Read the model definition and answer for the solid it produces. Units are mm, in the model's axes. Face numbers are marked on the shaded views. A direction names the side the tool comes from. Give positions to 0.01 mm unless a question says otherwise; leave off trailing zeros. Write each loop counter-clockwise with the first axis right and the second up, starting at its lowest first coordinate (ties: lowest second). Pieces come first, ordered by that corner, then holes. Notation, with made-up numbers: (-36.5, 77) -> (-29.5, 77) arc R21 cw to (-29.5, 95) -> close; hole circle Ø8 at (-29, 37.5). An arc over 180 degrees is marked (long way). Answer as CSV lines item,"result". Start each with the question number.
1. The part is cut by section C-C, the plane z = 0. Determine the outline of the cut face in (x, y), and give its area (3 significant figures).
2. Given pin 1 (2 mm diameter, centred on x = 22, z = 15, fed in from -Y); pin 2 (2.5 mm diameter, centred on y = 3, z = 0, fed in from +X); pin 3 (0.6 mm diameter, centred on y = -11, z = 8.5, fed in from -X), each flat-ended and moving along its own axis, determine where each tip first touches the part or whether it passes through.
3. Find the intervals of material crossed by line 1 (X direction, y = -4.75, z = 17); line 2 (Z direction, x = 1, y = -4.5); line 3 (Y direction, x = 18, z = 18), in increasing order.
4. A tool of negligible diameter and unlimited length cuts with its end or side. For the marked faces 1, 2, 3 and 4, from which of +Z, -Z, +X, -X, +Y, -Y can it reach the whole face along a straight path? Write none if from no direction.
5. The part is cut by section B-B, the plane y = -8.5. Determine the outline of the cut face in (x, z), and give its area (3 significant figures).
6. The part is cut by section A-A, the plane x = 0. Determine the outline of the cut face in (y, z).
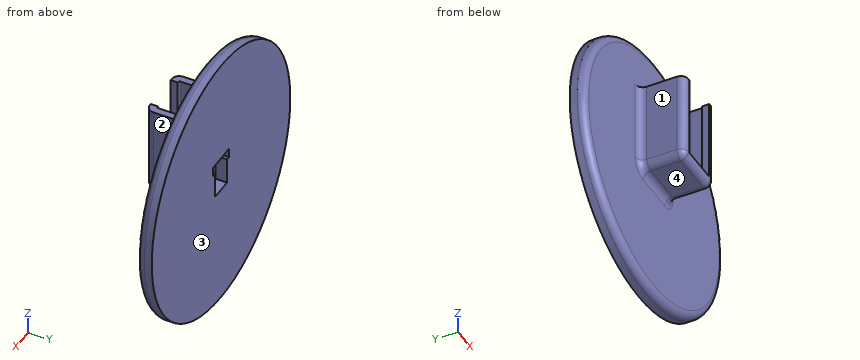
from build123d import *

# Parameters (mm, degrees)
SKETCH1_R                  = 35
ROUND_BODY_DEPTH           = 4
FILLET1_R                  = 2
SKETCH2_W                  = 6
SKETCH2_H                  = 7
SENSOR_SQUARE_HOLE_DEPTH   = 3
SKETCH4_W                  = 8
SKETCH4_H                  = 2.5
SENSOR_LEAD_HOLE_DEPTH     = 4
SKETCH5_W                  = 15
SKETCH5_H                  = 24
BACK_HOLDER_DEPTH          = 12
SKETCH6_W                  = 11.2
SKETCH6_H                  = 10.1
HOLDER_SLOT_DEPTH          = 22
HOLDER_ROUNDS_R            = 2
SKETCH7_W                  = 10
SKETCH7_H                  = 1.9
HOLDER_TOP_REMOVAL_DEPTH   = 22
HOLDER_MICRO_TOP_FILLETS_R = 0.5


with BuildPart() as part:
    # Sketch1 → Round Body (new body)
    with BuildSketch(Plane(origin=(0, 0, 0), x_dir=(1, 0, 0), z_dir=(0, 1, 0))):
        with Locations(Location((0, 0, 0), (0, 0, 270))):
            Circle(SKETCH1_R)
    extrude(amount=ROUND_BODY_DEPTH)

    # Fillet1
    fillet1_edges = [part.edges().sort_by_distance(p)[0] for p in [
        (0, 0, -35),
    ]]
    fillet(fillet1_edges, radius=FILLET1_R)

    # Sketch2 → Sensor Square Hole (cut)
    with BuildSketch(Plane(origin=(0, 4, 0), x_dir=(1, 0, 0), z_dir=(0, 1, 0))):
        with Locations((0, -1)):
            Rectangle(SKETCH2_W, SKETCH2_H)
    extrude(amount=-SENSOR_SQUARE_HOLE_DEPTH, mode=Mode.SUBTRACT)

    # Sketch4 → Sensor Lead Hole (cut)
    with BuildSketch(Plane(origin=(0, 4, 0), x_dir=(1, 0, 0), z_dir=(0, 1, 0))):
        with Locations((0, -5.75)):
            Rectangle(SKETCH4_W, SKETCH4_H)
    extrude(amount=-SENSOR_LEAD_HOLE_DEPTH, mode=Mode.SUBTRACT)

    # Sketch5 → Back Holder (add)
    with BuildSketch(Plane.XZ):
        with Locations((0, 9)):
            Rectangle(SKETCH5_W, SKETCH5_H)
    extrude(amount=BACK_HOLDER_DEPTH)

    # Sketch6 → Holder Slot (cut)
    with BuildSketch(Plane.XY.offset(21)):
        with Locations((0, -5.05)):
            Rectangle(SKETCH6_W, SKETCH6_H)
    extrude(amount=-HOLDER_SLOT_DEPTH, mode=Mode.SUBTRACT)

    # Holder Rounds
    holder_rounds_edges = [part.edges().sort_by_distance(p)[0] for p in [
        (-7.5, 0, 9),
        (0, 0, -3),
        (-7.5, -6, -3),
        (7.5, 0, 9),
        (7.5, -6, -3),
        (-7.5, -12, 9),
        (0, -12, -3),
        (7.5, -12, 9),
    ]]
    fillet(holder_rounds_edges, radius=HOLDER_ROUNDS_R)

    # Sketch7 → Holder Top Removal (cut)
    with BuildSketch(Plane.XY.offset(21)):
        with Locations((0, -11.05)):
            Rectangle(SKETCH7_W, SKETCH7_H)
    extrude(amount=-HOLDER_TOP_REMOVAL_DEPTH, mode=Mode.SUBTRACT)

    # Holder Micro Top fillets
    holder_micro_top_fillets_edges = [part.edges().sort_by_distance(p)[0] for p in [
        (-5.6, -10.1, 10),
        (5.6, -10.1, 10),
    ]]
    fillet(holder_micro_top_fillets_edges, radius=HOLDER_MICRO_TOP_FILLETS_R)


solid = part.part
Results found:
1,outline,"(-35, 2) arc R2 ccw to (-33, 0) -> (-9.5, 0) arc R2 cw to (-7.5, -2) -> (-7.5, -10) arc R2 ccw to (-5.5, -12) -> (-5, -12) -> (-5, -10.1) -> (-5.1, -10.1) arc R0.5 cw to (-5.6, -9.6) -> (-5.6, 0) -> (5.6, 0) -> (5.6, -9.6) arc R0.5 cw to (5.1, -10.1) -> (5, -10.1) -> (5, -12) -> (5.5, -12) arc R2 ccw to (7.5, -10) -> (7.5, -2) arc R2 cw to (9.5, 0) -> (33, 0) arc R2 ccw to (35, 2) -> (35, 4) -> (3, 4) -> (3, 1) -> (-3, 1) -> (-3, 4) -> (-35, 4) -> close"
1,area,"308 mm²"
2,pin 1,"stops at y = 0"
2,pin 2,"stops at x = 35"
2,pin 3,"stops at x = -7.37"
3,line 1,"x = -7.5 to -5.6, 5.6 to 7.5"
3,line 2,"z = -3 to -1"
3,line 3,"y = 0 to 4"
4,face 1,"+Z, -Z, -X, -Y"
4,face 2,"+Z, -Z, +X, -Y"
4,face 3,"+Z, -Z, +X, -X, +Y"
4,face 4,"-Z, +X, -X, -Y"
5,outline,"(-7.5, -1) arc R2 ccw to (-5.5, -3) -> (5.5, -3) arc R2 ccw to (7.5, -1) -> (7.5, 21) -> (5.6, 21) -> (5.6, -1) -> (-5.6, -1) -> (-5.6, 21) -> (-7.5, 21) -> close"
5,area,"112 mm²"
6,outline,"(-12, -1) arc R2 ccw to (-10, -3) -> (-2, -3) arc R2 cw to (0, -5) -> (0, -33) arc R2 ccw to (2, -35) -> (4, -35) -> (4, -2.5) -> (1, -2.5) -> (1, 4.5) -> (0, 4.5) -> (0, -1) -> close; (0, 7) -> (4, 7) -> (4, 35) -> (2, 35) arc R2 ccw to (0, 33) -> close"
